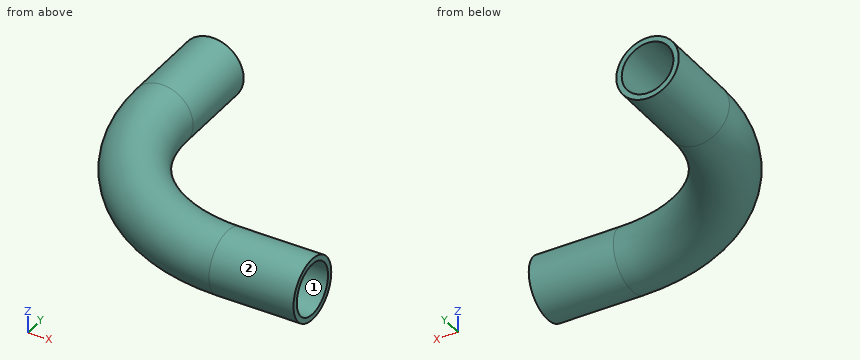
Autodesk Inventor part; units mm, degrees
ref_plane "YZ Plane" through (0, 0, 0) normal (1, 0, 0) x (0, 1, 0)
ref_plane "XZ Plane" through (0, 0, 0) normal (0, 1, 0) x (-1, 0, 0)
ref_plane "XY Plane" through (0, 0, 0) normal (0, 0, 1) x (1, 0, 0)
sketch "Sketch1" plane through (0, 0, 0) normal (0, 0, 1) x (1, 0, 0)
  line L0 (-76.7306, 50.268) -> (-77.0022, 76.2)
  line L1 (-25.9334, 0) -> (0, 0)
  arc A0 (-76.7306, 50.268) -> (-25.9334, 0) centre (-25.9334, 50.8) ccw
  dimension "d2" = 50.8
  dimension "d3" = 76.2
  dimension "d4" = 76.2
  dimension "d11" = 90.6
sketch "Sketch2" plane through (0, 0, 0) normal (1, 0, 0) x (0, 1, 0)
  circle A0 centre (0, 0) radius 9.525
  dimension "d7" = 19.05
sweep "Sweep1" add profiles "Sketch2" path "Sketch1"
shell "Shell1" thickness 1.65 removed faces 2 at (0, 1.5742, -0.5767) at (-73.9196, 76.2323, -0.7598)
equation "\"d2\" = 0.666667 * d4"
equation "\"d4\" = d3"
properties part number "90.6 DEG (ASME BPE) ELB-19.05"
Check sheet for the modelled part. Datum: model origin and axes. Units: mm. Face numbers are marked on the shaded views. Round coordinates to 2 decimals unless told otherwise and drop trailing zeros. Order: outer loops, then holes, each group sorted by start corner. A loop starts at its lowest first (then second) coordinate and runs counter-clockwise, first axis right, second up. Notation, with made-up numbers: M 18,-1 L 77,-1 A32 ccw 77,28 Z; hole C 19.5,44.25 d11. An arc over 180 degrees is marked long. Answer in a Markdown table with one row per item.
(1) Gauge pin test, flat ends, axial feed: pin 1 (10 mm diameter, centred on x = -20.5, y = 9.5, fed in from +Z) (3 decimals); pin 2 (6 mm diameter, centred on y = 19.5, z = -4.5, fed in from +X); pin 3 (10 mm diameter, centred on y = 51.5, z = -1, fed in from +X). Record the tip position at first contact, or that the pin passes through.
Findings:
| item | result |
|---|---|
| pin 1 | stops at z = 8.395 |
| pin 2 | stops at x = -50.29 |
| pin 3 | stops at x = -66.99 |
(2) Section check A-A on x = -23.5. Record the boundary of the cut face in (y, z) (3 decimals), plus the area to 3 significant figures.
Findings:
| item | result |
|---|---|
| outline | C 0,0 d19.05; hole C 0,0 d15.75 |
| area | 90.2 mm^2 |
(3) Material ranges on line 1 along Z through (x, y) = (-7, 0) (3 decimals); line 2 along X through (y, z) = (63, 6.5), recorded low to high. Write a range as from..to.
Findings:
| item | result |
|---|---|
| line 1 | z = -9.525..-7.875, 7.875..9.525 |
| line 2 | x = -83.83..-81.31, -72.42..-69.9 |
(4) Draft check along Y on the marked faces 1 and 2. Enter one of: +Y half, -Y half, draft (parallel to the pull), parting line (faces both ways), or undercut.
Findings:
| item | result |
|---|---|
| face 1 | undercut |
| face 2 | parting line |
